Part print with two shaded views. Sizes in mm from the minimum x, y, z corner. A direction names the side the tool comes from. Coordinates: 2 decimals unless noted, no trailing zeros. Loops run counter-clockwise (first coordinate to the right, second up) from the corner with the lowest first, then second, coordinate; pieces in that order, holes last.
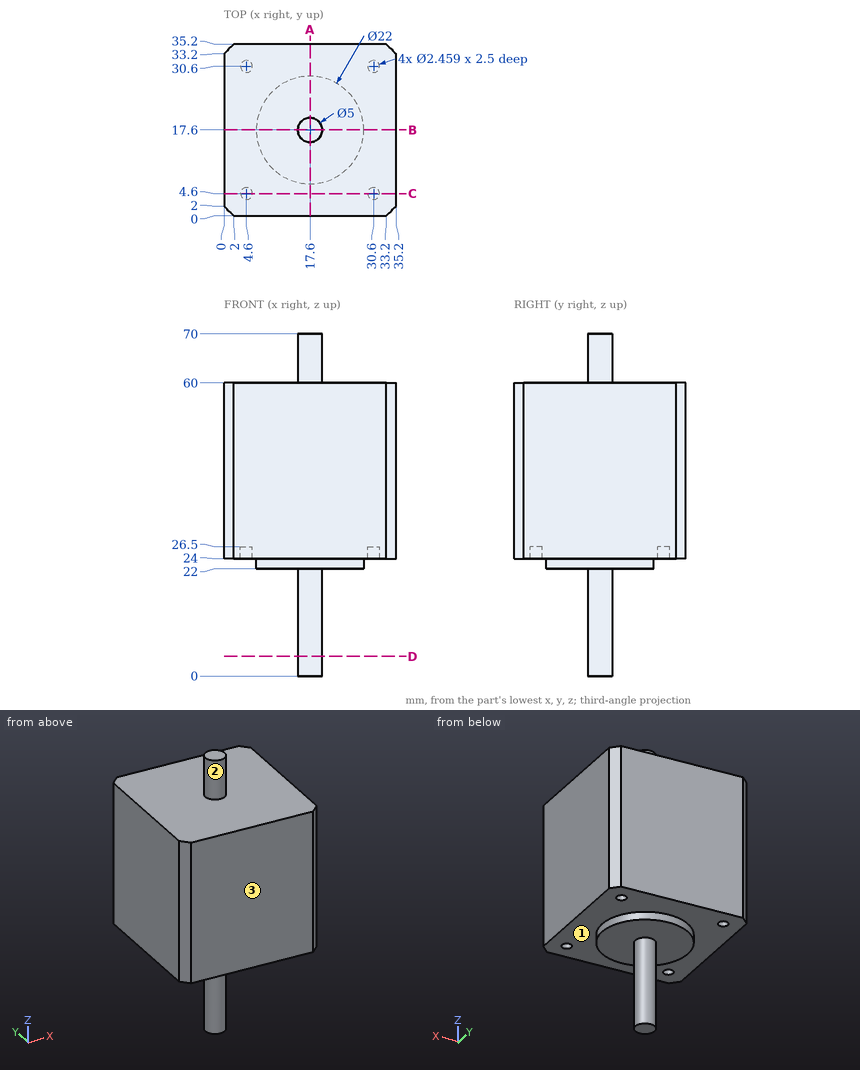
Q1. Drill centre lines: line 1 (Y direction, x = 30.6, z = 25); line 2 (Z direction, x = 9, y = 33.5). Where is each one in solid material? Low to high.
Answers:
line 1: y = 0 to 3.37, 5.83 to 29.37, 31.83 to 35.2
line 2: z = 24 to 60
Q2. Slice it at D-D (z = 4). List the corners of the cut face in (x, y).
Answers:
outline: circle Ø5 at (17.6, 17.6)
Q3. Slice it at A-A (x = 17.6). List the corners of the cut face in (y, z), and give its area (3 significant figures).
Answers:
outline: (0, 24) - (6.6, 24) - (6.6, 22) - (15.1, 22) - (15.1, 0) - (20.1, 0) - (20.1, 22) - (28.6, 22) - (28.6, 24) - (35.2, 24) - (35.2, 60) - (20.1, 60) - (20.1, 70) - (15.1, 70) - (15.1, 60) - (0, 60) - close
area: 1,470 mm2
Q4. Slice it at C-C (y = 4.6). List the corners of the cut face in (x, z).
Answers:
outline: (0, 24) - (3.37, 24) - (3.37, 26.5) - (5.83, 26.5) - (5.83, 24) - (29.37, 24) - (29.37, 26.5) - (31.83, 26.5) - (31.83, 24) - (35.2, 24) - (35.2, 60) - (0, 60) - close
Q5. Flat gauge pins, fed straight in: P1, Ø2, axis at x = 4.5, y = 30.5, coming from the -Z side; P2, Ø4, axis at x = 30.6, y = 4.6, coming from the -Z side; P3, Ø3, axis at x = 4.6, y = 30.6, coming from the +Z side; P4, Ø3, axis at x = 14, z = 47.5, coming from the -Y side. Where does each tip first touch, or does it go through?
Answers:
P1: stops at z = 26.5
P2: stops at z = 24
P3: stops at z = 60
P4: stops at y = 0
Q6. Which spindle directions (+Z, -Z, +X, -X, +Y, -Y) get a long thin tool onto all of the face, cutting with end or side? Do the marked faces 1, 2 and 3. Say none if no direction does.
Answers:
face 1: -Z
face 2: +Z
face 3: +Z, -Z, +X, -X, -Y
